Build history of the part. All positions in model axes, mm. Face numbers are marked on the shaded views. Give positions to 0.01 mm unless a question says otherwise; leave off trailing zeros. Order: outer loops, then holes, each group sorted by start corner. A loop starts at its lowest first (then second) coordinate and runs counter-clockwise, first axis right, second up. Notation, with made-up numbers: (51, 62.5) - (94, 62.5) arc R8 cw to (94, 74.5) - close; hole circle Ø10 at (27.25, -10.75). An arc over 180 degrees is marked (long way). Write each question's results on one line, items separated by ' | '. Start each with the question number.
1) Cut at A-A on z = 0. List the corners of the cut face in (x, y), plus the area to 3 significant figures.
2) Drill centre lines: line 1 along Y through (x, z) = (11.5, 0); line 2 along Z through (x, y) = (-3, 55.5); line 3 along Z through (x, y) = (0, 83). Where is each one in solid material? Low to high. Write a range as from..to.
3) Cut at B-B on x = 0. List the corners of the cut face in (y, z).
4) Cut at D-D on y = 62.5. List the corners of the cut face in (x, z), plus the area to 3 significant figures.
5) Two-plate mould, pull along Z, no slides. Class the marked faces 1, 2 and 3: +Z half, -Z half, draft (parallel to the pull), parting line (faces both ways), or undercut.
6) Cut at C-C on y = 6.5. List the corners of the cut face in (x, z).
7) Drop flat-ended pins along their axis: pin 1 Ø3.5 at (x, z) = (0, 0) entering from -Y; pin 2 Ø10.5 at (y, z) = (20.5, -30.5) entering from +X; pin 3 Ø10 at (y, z) = (57.5, -16) entering from -X; pin 4 Ø2 at (x, z) = (4.24, -4.24) entering from -Y. Give the stop position or say it passes through.
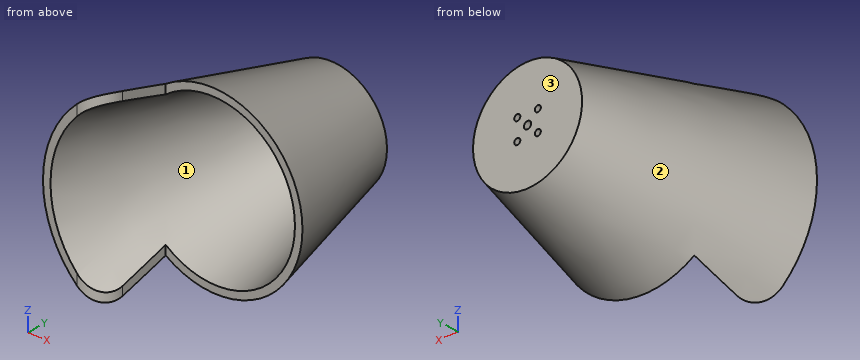
Autodesk Inventor part; units mm, degrees
ref_plane "YZ Plane" through (0, 0, 0) normal (1, 0, 0) x (0, 1, 0)
ref_plane "XZ Plane" through (0, 0, 0) normal (0, 1, 0) x (-1, 0, 0)
ref_plane "XY Plane" through (0, 0, 0) normal (0, 0, 1) x (1, 0, 0)
sketch "スケッチ8" plane through (0, 0, 0) normal (0, 0, 1) x (1, 0, 0)
  line L0 (0, 0) -> (0, 85)
  line L1 (0, 85) -> (22.5, 85)
  line L2 (22.5, 85) -> (44, 0)
  line L3 (44, 0) -> (0, 0)
  dimension "d14" = 22.5
  dimension "d15" = 44
  dimension "d16" = 85
revolve "回転1" add sketch "スケッチ8" angle 360 about axis through (0, 0, 0) along (0, 1, 0)
shell "シェル2" thickness 3 removed faces 1 at (-13.3987, 0, -0.1333)
sketch "スケッチ9" plane through (0, 82, 0) normal (0, -1, 0) x (1, 0, 0)
  circle A0 centre (0, 0) radius 1.5
  dimension "d29" = 3
hole "穴2" at (0, 82, 0) direction (0, 1, 0) diameter 3 end through all
sketch "スケッチ16" plane through (0, 0, 0) normal (0, -1, 0) x (1, 0, 0)
  line L0 (80, -50) -> (-20, -50)
  line L1 (-20, -50) -> (-20, 50)
  line L2 (-20, 50) -> (80, 50)
  line L3 (80, 50) -> (80, -50)
  point P0 (0, 0)
  dimension "d66" = 100
  dimension "d67" = 100
  dimension "d68" = 50
  dimension "d69" = 20
extrude "押し出し6" cut sketch "スケッチ16" against normal blind 30
fillet "フィレット3" radius 10 2 edges at (-20, 0, -37.4373) (-20, 0, 37.4373)
sketch "スケッチ17" plane through (0, 82, 0) normal (0, -1, 0) x (1, 0, 0)
  line L0 (0, 0) -> (-4.2426, -4.2426)
  line L1 (0, 0) -> (6, 0) construction
  circle A0 centre (-4.2426, -4.2426) radius 1.25
  dimension "d73" = 6
  dimension "d74" = 135
  dimension "d75" = 2.5
extrude "押し出し7" cut sketch "スケッチ17" against normal blind 30
pattern_circular "円形状パターン2" count 4 over 360 about axis through (0, 232.7083, 0) along (0, -1, 0) of "押し出し7"
properties part number "ball受け" material "ABS プラスチック"
Results:
1) outline: (-44, 0) - (-40.91, 0) - (-20.16, 82) - (-1.5, 82) - (-1.5, 85) - (-22.5, 85) - close; (1.5, 82) - (20.16, 82) - (33.32, 30) - (36.41, 30) - (22.5, 85) - (1.5, 85) - close | area: 543 mm^2
2) line 1: 82..85 | line 2: -29.81..-26.7, 26.7..29.81 | line 3: -23.01..-1.5, 1.5..23.01
3) outline: (30, -36.41) - (85, -22.5) - (85, -1.5) - (82, -1.5) - (82, -20.16) - (30, -33.32) - close; (30, 33.32) - (82, 20.16) - (82, 1.5) - (85, 1.5) - (85, 22.5) - (30, 36.41) - close
4) outline: circle Ø56.38 at (0, 0); hole circle Ø50.19 at (0, 0) | area: 518 mm^2
5) face 1: undercut | face 2: parting line | face 3: draft
6) outline: (-20.63, -36.99) - (-20.63, -33.4) arc R39.26 cw to (-20.63, 33.4) - (-20.63, 36.99) arc R42.36 ccw to start
7) pin 1: y = 82 | pin 2: x = -20 | pin 3: x = -27.74 | pin 4: through
